For this review, use the dimensioned drawing (mm, ordinates from the lowest corner) and the shaded views. A direction names the side the tool comes from. Round coordinates to 2 decimals unless told otherwise and drop trailing zeros. Write each loop counter-clockwise with the first axis right and the second up, starting at its lowest first coordinate (ties: lowest second). Pieces come first, ordered by that corner, then holes. Notation, with made-up numbers: (-12.75, -26) - (15.25, -26) arc R30 ccw to (15.25, -2) - close; hole circle Ø2 at (7, 73). An arc over 180 degrees is marked (long way). Write each question's results on one line, items separated by ' | '.
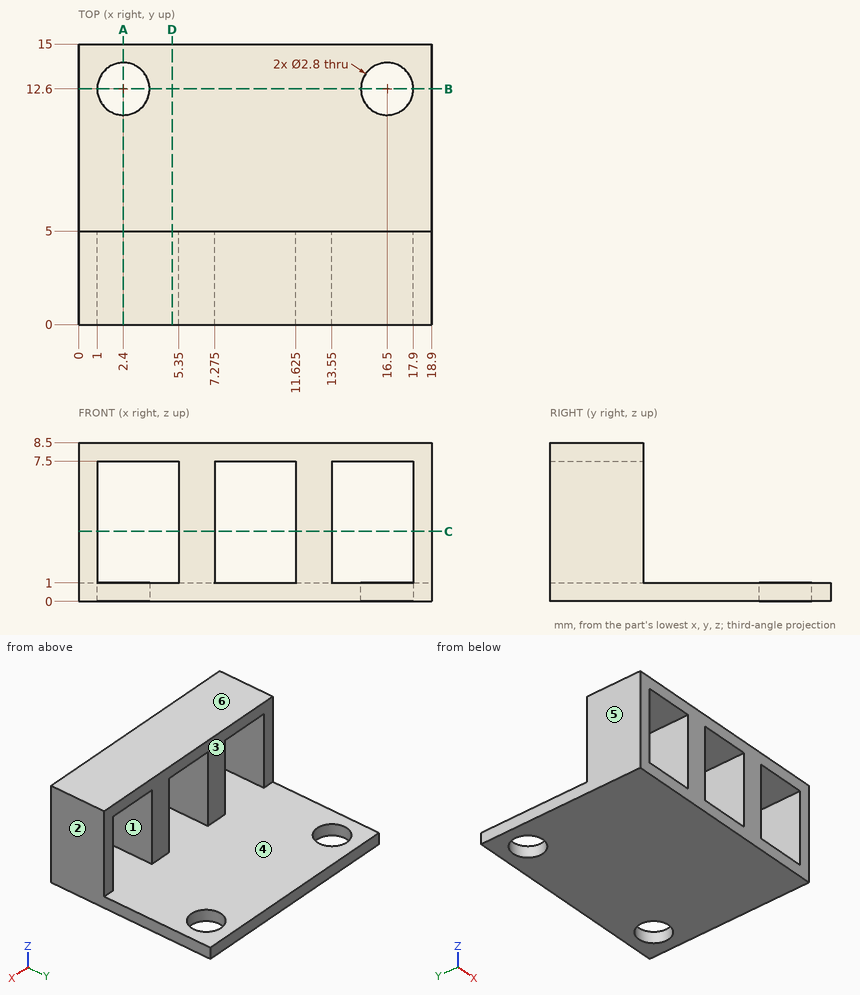
Q1. Tool access review of the marked faces 1, 2 and 3: name each direction out of +Z, -Z, +X, -X, +Y, -Y from which nothing blocks a thin tool from reaching the whole face with its end or side.
Evaluation:
face 1: +Y, -Y | face 2: +Z, -Z, +X, +Y, -Y | face 3: +Z, +X, -X, +Y
Q2. Insertion check: P1, Ø2, axis at x = 16.5, y = 12.6, coming from the -Z side; P2, Ø3.5, axis at x = 2.4, y = 12.6, coming from the +Z side. Each pin has a flat end and moves straight along its axis. Give the tip position at first contact, or say it passes through.
Evaluation:
P1: passes through | P2: stops at z = 1
Q3. For probe 1 along X at (y, z) = (1.5, 7) (3 decimals); probe 2 along Y at (x, z) = (2.4, 0.3); probe 3 along Z at (x, y) = (9.25, 2), list the stretches that pass through material, from the lowest coordinate up.
Evaluation:
probe 1: x = 0 to 1, 5.35 to 7.275, 11.625 to 13.55, 17.9 to 18.9 | probe 2: y = 0 to 11.2, 14 to 15 | probe 3: z = 0 to 1, 7.5 to 8.5
Q4. We need section B-B (y = 12.6). State the section outline as (x, z) points, plus the area to 3 significant figures.
Evaluation:
outline: (0, 0) - (1, 0) - (1, 1) - (0, 1) - close; (3.8, 0) - (15.1, 0) - (15.1, 1) - (3.8, 1) - close; (17.9, 0) - (18.9, 0) - (18.9, 1) - (17.9, 1) - close | area: 13.3 mm^2
Q5. The part is to be moulded in two halves that separate along X. For the marked faces 4, 5 and 6, say which applies: released by +X, released by -X, zero draft, split by the parting line, or undercut.
Evaluation:
face 4: undercut | face 5: released by -X | face 6: zero draft
Q6. We need section A-A (x = 2.4). State the section outline as (y, z) points.
Evaluation:
outline: (0, 0) - (11.2, 0) - (11.2, 1) - (0, 1) - close; (0, 7.5) - (5, 7.5) - (5, 8.5) - (0, 8.5) - close; (14, 0) - (15, 0) - (15, 1) - (14, 1) - close
Q7. We need section D-D (x = 5). State the section outline as (y, z) points.
Evaluation:
outline: (0, 0) - (15, 0) - (15, 1) - (0, 1) - close; (0, 7.5) - (5, 7.5) - (5, 8.5) - (0, 8.5) - close
Q8. We need section C-C (z = 3.75). State the section outline as (x, y) points (3 decimals).
Evaluation:
outline: (0, 0) - (1, 0) - (1, 5) - (0, 5) - close; (5.35, 0) - (7.275, 0) - (7.275, 5) - (5.35, 5) - close; (11.625, 0) - (13.55, 0) - (13.55, 5) - (11.625, 5) - close; (17.9, 0) - (18.9, 0) - (18.9, 5) - (17.9, 5) - close
